Can you work these out from the drawing? Everything is in mm from the part's minimum corner. A direction names the side the tool comes from. Coordinates: 2 decimals unless noted, no trailing zeros. Loops run counter-clockwise (first coordinate to the right, second up) from the corner with the lowest first, then second, coordinate; pieces in that order, holes last.
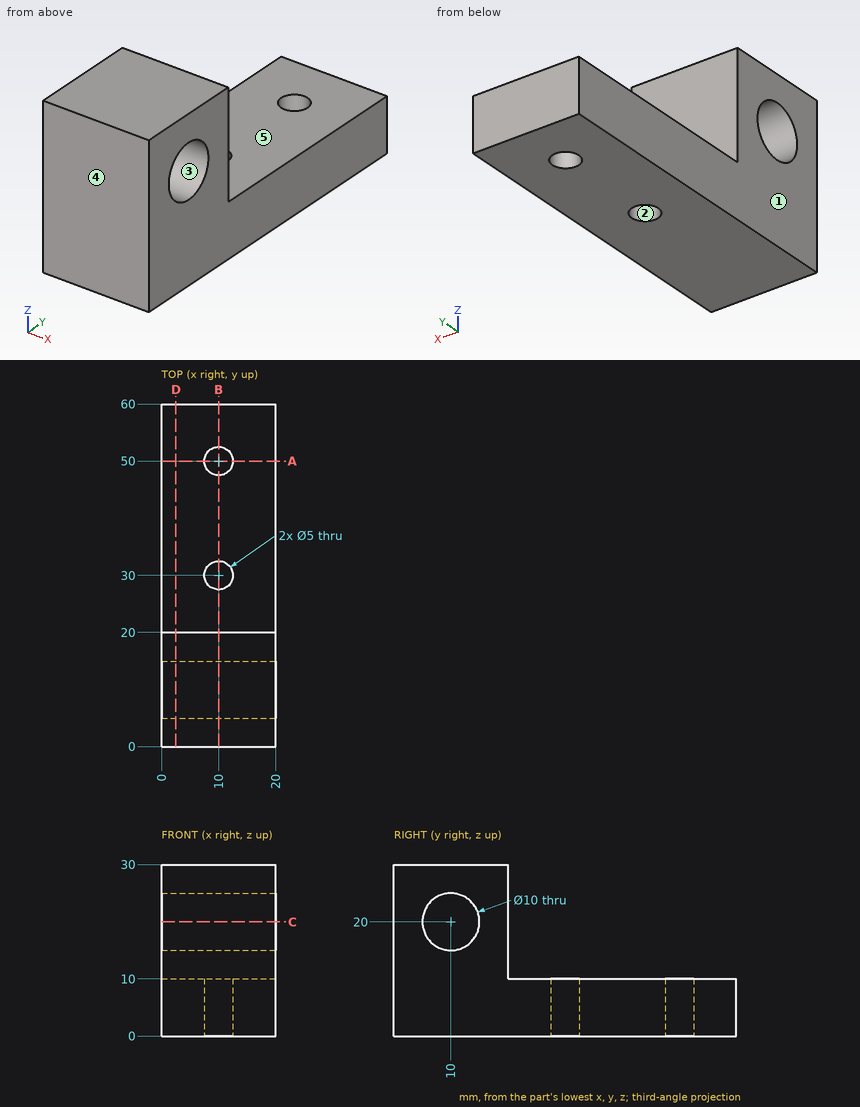
(1) Imagine slicing it at B-B, the plane x = 10. Write out the boundary of the cut face in (y, z).
Answers:
outline: (0, 0) - (27.5, 0) - (27.5, 10) - (20, 10) - (20, 30) - (0, 30) - close; (32.5, 0) - (47.5, 0) - (47.5, 10) - (32.5, 10) - close; (52.5, 0) - (60, 0) - (60, 10) - (52.5, 10) - close; hole circle Ø10 at (10, 20)
(2) Imagine slicing it at A-A, the plane y = 50. Write out the boundary of the cut face in (x, z), and give its area (3 significant figures).
Answers:
outline: (0, 0) - (7.5, 0) - (7.5, 10) - (0, 10) - close; (12.5, 0) - (20, 0) - (20, 10) - (12.5, 10) - close
area: 150 mm2
(3) Imagine slicing it at C-C, the plane z = 20. Write out the boundary of the cut face in (x, y).
Answers:
outline: (0, 0) - (20, 0) - (20, 5) - (0, 5) - close; (0, 15) - (20, 15) - (20, 20) - (0, 20) - close
(4) For pin 1 (8 mm diameter, centred on x = 16.5, z = 23.5, fed in from +Y); pin 2 (4 mm diameter, centred on x = 10, y = 50, fed in from -Z); pin 3 (6 mm diameter, centred on x = 11.5, y = 31, fed in from +Z), each with a flat end and sliding along its axis, tell me the tip position at first contact or that it passes through.
Answers:
pin 1: stops at y = 20
pin 2: passes through
pin 3: stops at z = 10
(5) Imagine slicing it at D-D, the plane x = 2.5. Write out the boundary of the cut face in (y, z), and give its area (3 significant figures).
Answers:
outline: (0, 0) - (60, 0) - (60, 10) - (20, 10) - (20, 30) - (0, 30) - close; hole circle Ø10 at (10, 20)
area: 921 mm2
(6) Which directions (+Z, -Z, +X, -X, +Y, -Y) give clear straight access to the entire face, cutting with the end or side of a thin tool? Please do the marked faces 4 and 5.
Answers:
face 4: +Z, -Z, +X, -X, -Y
face 5: +Z, +X, -X, +Y
(7) I need wall thicknesses on probe 1 along Y at (x, z) = (10, 7.75); probe 2 along Y at (x, z) = (1.5, 25.75); probe 3 along Y at (x, z) = (8, 9.5). Which ranges of each line are inside material? Lowest first, please.
Answers:
probe 1: y = 0 to 27.5, 32.5 to 47.5, 52.5 to 60
probe 2: y = 0 to 20
probe 3: y = 0 to 28.5, 31.5 to 48.5, 51.5 to 60
(8) We'd pull the mould along X, two halves only. Please class the marked faces 1, 2 and 3: +X half, -X half, draft (parallel to the pull), parting line (faces both ways), or undercut.
Answers:
face 1: -X half
face 2: undercut
face 3: draft
